from build123d import *

# Parameters (mm, degrees)
SKETCH_3_W          = 24
SKETCH_3_H          = 8
CUT_EXTRUDE_1_DEPTH = 28
SKETCH_4_W          = 16
SKETCH_4_H          = 32
EXTRUDE_1_DEPTH     = 2
SKETCH_5_R          = 1.5
EXTRUDE_2_DEPTH     = 20
SKETCH_6_R          = 1.5
CUT_EXTRUDE_2_DEPTH = 77.229915477


with BuildPart() as part:
    # 草图2 → 放样1 section 0
    with BuildSketch(Plane(origin=(31, 0, 0), x_dir=(0, 0, -1), z_dir=(1, 0, 0))):
        with BuildLine():
            Line((-37, 31), (37, 31))
            Line((37, 31), (37, -31))
            Line((37, -31), (-37, -31))
            Line((-37, -31), (-37, 31))
        make_face()
    # 草图1 → 放样1 section 1
    with BuildSketch(Plane(origin=(0, 0, 0), x_dir=(0, 0, -1), z_dir=(1, 0, 0))):
        with BuildLine():
            Line((-37, 37), (37, 37))
            Line((37, 37), (37, -37))
            Line((37, -37), (-37, -37))
            Line((-37, -37), (-37, 37))
        make_face()
    loft()

    # 草图3 → 切除-拉伸1 (cut)
    with BuildSketch(Plane(origin=(31, 0, 0), x_dir=(0, 0, -1), z_dir=(1, 0, 0))):
        with Locations((0, 33)):
            Rectangle(SKETCH_3_W, SKETCH_3_H)
    cut_extrude_1 = extrude(amount=-CUT_EXTRUDE_1_DEPTH, mode=Mode.SUBTRACT)

    # 镜向1: 切除-拉伸1 across plane
    add(cut_extrude_1.mirror(Plane.ZX), mode=Mode.SUBTRACT)

    # 草图4 → 凸台-拉伸1 (add)
    with BuildSketch(Plane.XY.offset(37)):
        with Locations((8, 0)):
            Rectangle(SKETCH_4_W, SKETCH_4_H)
    extrude(amount=EXTRUDE_1_DEPTH)

    # 草图5 → 凸台-拉伸2 (add)
    with BuildSketch(Plane.XY.offset(39)):
        with Locations(Location((5, -3, 0), (0, 0, 180))):
            Circle(SKETCH_5_R)
        with Locations(Location((5, -9, 0), (0, 0, 180))):
            Circle(SKETCH_5_R)
    extrude_2 = extrude(amount=EXTRUDE_2_DEPTH)

    # 镜向2: 凸台-拉伸2 across plane
    add(extrude_2.mirror(Plane.ZX))

    # 草图6 → 切除-拉伸2 (cut, through all)
    with BuildSketch(Plane.ZY):
        with Locations((0, -32.5)):
            Circle(SKETCH_6_R)
    cut_extrude_2 = extrude(amount=-CUT_EXTRUDE_2_DEPTH, mode=Mode.SUBTRACT)

    # 镜向3: 切除-拉伸2 across plane
    add(cut_extrude_2.mirror(Plane.ZX), mode=Mode.SUBTRACT)


solid = part.part
Geometry: final body of the model. Coordinates: model frame, mm. A direction names the side the tool comes from. Give positions to 0.01 mm unless a question says otherwise; leave off trailing zeros. Write each loop counter-clockwise with the first axis right and the second up, starting at its lowest first coordinate (ties: lowest second). Pieces come first, ordered by that corner, then holes. Notation, with made-up numbers: M -36,66 L 2,66 A31 ccw 2,105 Z; hole C -22,-32.5 d5. An arc over 180 degrees is marked long. Answer in a Markdown table with one row per item. Add a question column.
(1) Ray query, line 1 (Z direction, x = 17, y = -31); line 2 (Y direction, x = 1.55, z = 0); line 3 (Y direction, x = 0.7, z = 0). Return the intervals inside material, ascending.
(2) First-contact query: pin 1 (1 mm diameter, centred on y = -8.5, z = 3, fed in from -X); pin 2 (1 mm diameter, centred on x = 9.5, z = 38.5, fed in from -Y); pin 3 (8 mm diameter, centred on x = 24, y = -33, fed in from +Z); pin 4 (2.5 mm diameter, centred on y = -32.5, z = 0, fed in from -X). Flat tips, straight axial feed; report the tip coordinate or a pass-through.
(3) Section A-A on z = 0. Return loops of the section in (x, y), and give its area (3 significant figures).
(4) Reachability of faces 5 (the cylindrical face through (5.325, -7.536, 48.86)), 6 (the flat face through (17, 29, 0)), 7 (the flat face through (16, 0, 38)), 8 (the flat face through (8, -16, 38)) from +Z, -Z, +X, -X, +Y, -Y: full face, straight path, thin tool, end or side. Return the list, or none.
(5) Section B-B on z = -27.5. Return loops of the section in (x, y).
(6) Mould query, pull axis Y, two halves, no side actions, for faces 1 (the cylindrical face through (6.2, -2.1, 48.9)), 2 (the flat face through (3, -34.4, 0.2)), 3 (the flat face through (8, 16, 38)), 4 (the cylindrical face through (1, -34, 0)). Classes: +Y half, -Y half, draft (parallel to the pull), parting line (faces both ways), or undercut.
Result set:
| question | item | result |
|---|---|---|
| 1 | line 1 | z = -37 to -12, 12 to 37 |
| 1 | line 2 | y = -36.7 to -34, -31 to 31, 34 to 36.7 |
| 1 | line 3 | y = -36.86 to -34, -31 to 31, 34 to 36.86 |
| 2 | pin 1 | stops at x = 0 |
| 2 | pin 2 | stops at y = -16 |
| 2 | pin 3 | stops at z = 37 |
| 2 | pin 4 | passes through |
| 3 | outline | M 0,-37 L 3,-36.42 L 3,-34 L 0,-34 Z; M 0,-31 L 3,-31 L 3,-29 L 31,-29 L 31,29 L 3,29 L 3,31 L 0,31 Z; M 0,34 L 3,34 L 3,36.42 L 0,37 Z |
| 3 | area | 1,830 mm^2 |
| 4 | face 5 | +Z |
| 4 | face 6 | +X, +Y |
| 4 | face 7 | +Z, +X, +Y, -Y |
| 4 | face 8 | +Z, +X, -X, -Y |
| 5 | outline | M 0,-37 L 31,-31 L 31,31 L 0,37 Z |
| 6 | face 1 | undercut |
| 6 | face 2 | draft |
| 6 | face 3 | +Y half |
| 6 | face 4 | undercut |
